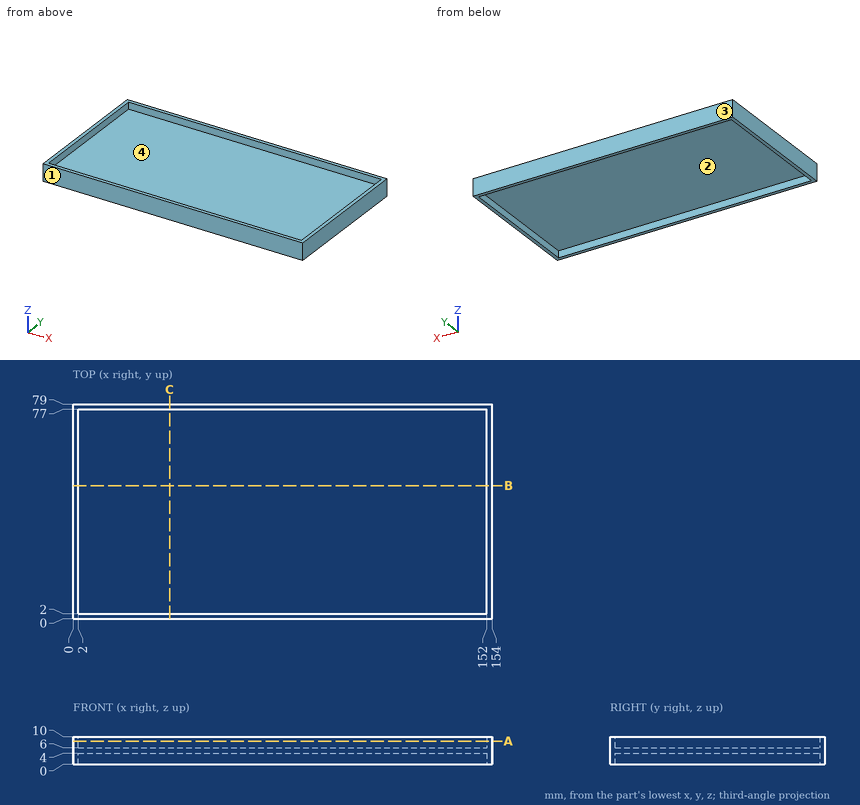
For this review, use the dimensioned drawing (mm, ordinates from the lowest corner) and the shaded views. A direction names the side the tool comes from. Give positions to 0.01 mm unless a question says otherwise; leave off trailing zeros. Write each loop counter-clockwise with the first axis right and the second up, starting at its lowest first coordinate (ties: lowest second). Pieces come first, ordered by that corner, then holes. Notation, with made-up numbers: M 25.5,57.25 L 80.5,57.25 A19 cw 80.5,88.25 Z; hole C 86,-32 d6. An arc over 180 degrees is marked long. Answer as a JSON object with one key per item and string values. Group by question number.
1) We need section A-A (z = 8.5). Give the boundary of the cut face in (x, y), and give its area (3 significant figures).
2) For line 1 along Y through (x, z) = (76.5, 3); line 2 along X through (y, z) = (44, 9); line 3 along Z through (x, y) = (86, 40), list the stretches that pass through material, from the lowest coordinate up.
3) Tool access review of the marked faces 1 and 2: name each direction out of +Z, -Z, +X, -X, +Y, -Y from which nothing blocks a thin tool from reaching the whole face with its end or side.
4) We need section C-C (x = 35.5). Give the boundary of the cut face in (y, z), and give its area (3 significant figures).
5) Clearance check with flat-ended pins moving along their axes: pin 1 Ø5 at (x, y) = (72, 35.5) entering from +Z; pin 2 Ø2 at (x, z) = (109.5, 8.5) entering from -Y; pin 3 Ø4 at (x, y) = (88.5, 17.5) entering from -Z. State where each tip first meets the part, or that it passes through.
6) We need section B-B (y = 49). Give the boundary of the cut face in (x, z), and give its area (3 significant figures).
7) Mouldability with a two-part tool opening along X and no side actions: class the marked faces 3 and 4 as released by +X, released by -X, zero draft, split by the parting line, or undercut.
Answer key:
{
 "1": {"outline": "M 0,0 L 154,0 L 154,79 L 0,79 Z; hole M 2,2 L 152,2 L 152,77 L 2,77 Z", "area": "916 mm²"},
 "2": {"line 1": "y = 0 to 2, 77 to 79", "line 2": "x = 0 to 2, 152 to 154", "line 3": "z = 4 to 6"},
 "3": {"face 1": "+Z, -Z, +X, -X, -Y", "face 2": "-Z"},
 "4": {"outline": "M 0,0 L 2,0 L 2,4 L 77,4 L 77,0 L 79,0 L 79,10 L 77,10 L 77,6 L 2,6 L 2,10 L 0,10 Z", "area": "190 mm²"},
 "5": {"pin 1": "stops at z = 6", "pin 2": "stops at y = 0", "pin 3": "stops at z = 4"},
 "6": {"outline": "M 0,0 L 2,0 L 2,4 L 152,4 L 152,0 L 154,0 L 154,10 L 152,10 L 152,6 L 2,6 L 2,10 L 0,10 Z", "area": "340 mm²"},
 "7": {"face 3": "zero draft", "face 4": "undercut"}
}
